The model under review builds one solid part; all positions refer to its coordinate system, in mm. Give positions to 0.01 mm unless a question says otherwise; leave off trailing zeros. Write each loop counter-clockwise with the first axis right and the second up, starting at its lowest first coordinate (ties: lowest second). Pieces come first, ordered by that corner, then holes. Notation, with made-up numbers: (11, 52.5) -> (64, 52.5) arc R21 ccw to (64, 62.5) -> close; hole circle Ø4 at (3, -10.5). An arc over 180 degrees is marked (long way). Use CSV: the item, a comma, the result in double quotes.
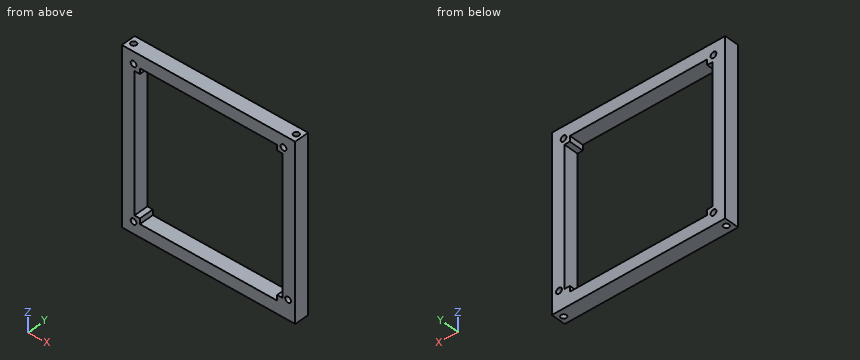
```python
from build123d import *

# Parameters (mm, degrees)
SKETCH1_W                    = 96
SKETCH1_H                    = 96
SKETCH1_W_2                  = 80
SKETCH1_H_2                  = 80
BOSS_EXTRUDE1_DEPTH          = 8
F_3_0_3_DIAMETER_HOLE6_D     = 3
F_3_0_3_DIAMETER_HOLE6_DEPTH = 6
F_3_0_3_DIAMETER_HOLE3_D     = 3
F_3_0_3_DIAMETER_HOLE3_DEPTH = 6
SKETCH27_W                   = 82
SKETCH27_H                   = 82
CUT_EXTRUDE2_DEPTH           = 10
SKETCH35_W                   = 3
SKETCH35_H                   = 3
BOSS_EXTRUDE2_DEPTH          = 8
F_3_2_3_2_DIAMETER_HOLE1_D   = 3.2


with BuildPart() as part:
    # Sketch1 → Boss-Extrude1 (new body)
    with BuildSketch(Plane(origin=(0, 0, 0), x_dir=(1, 0, 0), z_dir=(0, 1, 0))):
        Rectangle(SKETCH1_W, SKETCH1_H)
        Rectangle(SKETCH1_W_2, SKETCH1_H_2, mode=Mode.SUBTRACT)
    extrude(amount=BOSS_EXTRUDE1_DEPTH)

    # Ø3.0 (3) Diameter Hole6
    with Locations(Plane.XY.offset(48)):
        with Locations((45, 4), (-45, 4)):
            Hole(F_3_0_3_DIAMETER_HOLE6_D / 2, depth=F_3_0_3_DIAMETER_HOLE6_DEPTH)

    # Ø3.0 (3) Diameter Hole3
    with Locations(Plane(origin=(0, 0, -48), x_dir=(-1, 0, 0), z_dir=(0, 0, -1))):
        with Locations((45, 4), (-45, 4)):
            Hole(F_3_0_3_DIAMETER_HOLE3_D / 2, depth=F_3_0_3_DIAMETER_HOLE3_DEPTH)

    # Sketch27 → Cut-Extrude2 (cut)
    with BuildSketch(Plane(origin=(0, 8, 0), x_dir=(1, 0, 0), z_dir=(0, 1, 0))):
        Rectangle(SKETCH27_W, SKETCH27_H)
    extrude(amount=-CUT_EXTRUDE2_DEPTH, mode=Mode.SUBTRACT)

    # Sketch35 → Boss-Extrude2 (add)
    with BuildSketch(Plane(origin=(0, 8, 0), x_dir=(1, 0, 0), z_dir=(0, 1, 0))):
        with Locations((-39.5, 39.5)):
            Rectangle(SKETCH35_W, SKETCH35_H)
        with Locations((39.5, 39.5)):
            Rectangle(SKETCH35_W, SKETCH35_H)
        with Locations((39.5, -39.5)):
            Rectangle(SKETCH35_W, SKETCH35_H)
        with Locations((-39.5, -39.5)):
            Rectangle(SKETCH35_W, SKETCH35_H)
    extrude(amount=-BOSS_EXTRUDE2_DEPTH)

    # Ø3.2 (3.2) Diameter Hole1 (through all)
    with Locations(Plane(origin=(0, 8, 0), x_dir=(1, 0, 0), z_dir=(0, 1, 0))):
        with Locations((44.05, 37.33), (41.5, -41.5), (-41.5, -41.5), (-41.5, 41.5)):
            Hole(F_3_2_3_2_DIAMETER_HOLE1_D / 2)


solid = part.part
```
Q1. Consider section C-C (x = -45). Write out the cut boundary in (y, z).
Derived:
outline,"(0, -48) -> (2.5, -48) -> (2.5, -42) -> (5.5, -42) -> (5.5, -48) -> (8, -48) -> (8, 48) -> (5.5, 48) -> (5.5, 42) -> (2.5, 42) -> (2.5, 48) -> (0, 48) -> close"
Q2. To check wall thickness, follow probe 1 along Z at (x, y) = (-41.5, 4.25); probe 2 along Z at (x, y) = (-19.5, 2). State the ranges of each line that lie inside material, in increasing order.
Derived:
probe 1,"z = -48 to -43.1, -39.9 to 39.9, 43.1 to 48"
probe 2,"z = -48 to -41, 41 to 48"
Q3. Consider section B-B (z = -26). Write out the cut boundary in (x, y), then the cut area to 3 significant figures.
Derived:
outline,"(-48, 0) -> (-41, 0) -> (-41, 8) -> (-48, 8) -> close; (41, 0) -> (48, 0) -> (48, 8) -> (41, 8) -> close"
area,"112 mm2"
Q4. Insertion check: pin 1 (2.5 mm diameter, centred on x = -45, y = 4, fed in from -Z); pin 2 (3 mm diameter, centred on x = 41.5, z = 41.5, fed in from +Y). Each pin has a flat end and moves straight along its axis. Give the tip position at first contact, or say it passes through.
Derived:
pin 1,"stops at z = -42"
pin 2,"passes through"
Q5. Consider section A-A (x = 19.5). Write out the cut boundary in (y, z).
Derived:
outline,"(0, -48) -> (8, -48) -> (8, -41) -> (0, -41) -> close; (0, 41) -> (8, 41) -> (8, 48) -> (0, 48) -> close"
